For this review, take the finished solid that the model builds, in its own axes (mm). Face numbers are marked on the shaded views. A direction names the side the tool comes from. Coordinates: 2 decimals unless noted, no trailing zeros. Write each loop counter-clockwise with the first axis right and the second up, starting at its lowest first coordinate (ties: lowest second). Pieces come first, ordered by that corner, then holes. Notation, with made-up numbers: M -2,19.5 L 46,19.5 A28 ccw 46,44.5 Z; hole C 61.5,66 d4. An arc over 180 degrees is marked long. One line per question, with ' | ' between items.
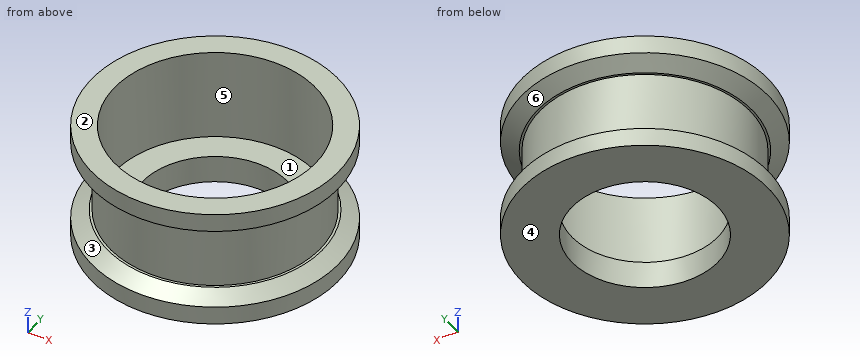
from build123d import *

# Parameters (mm, degrees)
SKETCH1_R           = 13.5
SKETCH1_R_2         = 8
BOSS_EXTRUDE1_DEPTH = 13
SKETCH2_R           = 11
CUT_EXTRUDE1_DEPTH  = 10
CUT_EXTRUDE2_START  = -3
SKETCH3_OUTSIDE_W   = 37.068
SKETCH3_OUTSIDE_H   = 37.068
SKETCH3_OUTSIDE_R   = 11.5
CUT_EXTRUDE2_DEPTH  = 7
CHAMFER1_SIZE       = 1.75
CHAMFER1_SIZE2      = 1.010362971
CHAMFER2_SIZE       = 1
CHAMFER2_SIZE2      = 1.732050808


with BuildPart() as part:
    # Sketch1 → Boss-Extrude1 (new body)
    with BuildSketch(Plane.XY):
        Circle(SKETCH1_R)
        Circle(SKETCH1_R_2, mode=Mode.SUBTRACT)
    extrude(amount=BOSS_EXTRUDE1_DEPTH)

    # Sketch2 → Cut-Extrude1 (cut)
    with BuildSketch(Plane.XY.offset(13)):
        Circle(SKETCH2_R)
    extrude(amount=-CUT_EXTRUDE1_DEPTH, mode=Mode.SUBTRACT)

    # Sketch3 outside → Cut-Extrude2 (cut)
    with BuildSketch(Plane.XY.offset(13).offset(CUT_EXTRUDE2_START)):
        Rectangle(SKETCH3_OUTSIDE_W, SKETCH3_OUTSIDE_H)
        Circle(SKETCH3_OUTSIDE_R, mode=Mode.SUBTRACT)
    extrude(amount=-CUT_EXTRUDE2_DEPTH, mode=Mode.SUBTRACT)

    # Chamfer1
    chamfer1_edges = [part.edges().sort_by_distance(p)[0] for p in [
        (-13.5, 0, 10),
    ]]
    chamfer1_side = [part.faces().sort_by_distance(p)[0] for p in [
        (-13.118162338, 0, 10),
    ]]
    chamfer(chamfer1_edges, length=CHAMFER1_SIZE, length2=CHAMFER1_SIZE2, reference=chamfer1_side[0])

    # Chamfer2
    chamfer2_edges = [part.edges().sort_by_distance(p)[0] for p in [
        (-13.5, 0, 3),
    ]]
    chamfer2_side = [part.faces().sort_by_distance(p)[0] for p in [
        (-13.5, 0, 1.5),
    ]]
    chamfer(chamfer2_edges, length=CHAMFER2_SIZE, length2=CHAMFER2_SIZE2, reference=chamfer2_side[0])


solid = part.part
1. Take a section at C-C on z = 4.5. State the section outline as (x, y) points.
Computed values:
outline: C 0,0 d23; hole C 0,0 d22
2. Machinability: for the marked faces 4, 5 and 6, which of the approach directions +Z, -Z, +X, -X, +Y, -Y give a long, thin tool a straight path to every point of the face, cutting with its end or side? Answer none if there is none.
Computed values:
face 4: -Z, +X, -X, +Y, -Y | face 5: +Z | face 6: none
3. Draft analysis for pull direction X (two halves, no side actions). For the marked faces 1, 2 and 3, state which applies: pulls with the +X half, pulls with the -X half, needs draft (parallel to the pull), parting line crosses it, or undercut.
Computed values:
face 1: undercut | face 2: needs draft | face 3: parting line crosses it
4. For line 1 along X through (y, z) = (0, 0.8); line 2 along Y through (x, z) = (0.25, 11.5), list the stretches that pass through material, from the lowest coordinate up.
Computed values:
line 1: x = -13.5 to -8, 8 to 13.5 | line 2: y = -13.5 to -11, 11 to 13.5
5. Clearance check with flat-ended pins moving along their axes: P1, Ø1, axis at x = -2.5, z = 4.5, coming from the +Y side; P2, Ø2, axis at x = -5.5, y = 3, coming from the -Z side; P3, Ø12, axis at x = 4, y = -5, coming from the -Z side; P4, Ø2, axis at y = -9, z = 8, coming from the +X side. State where each tip first meets the part, or that it passes through.
Computed values:
P1: stops at y = 11.32 | P2: passes through | P3: stops at z = 0 | P4: stops at x = 8.26
6. Take a section at A-A on x = 0. State the section outline as (y, z) points.
Computed values:
outline: M -13.5,0 L -8,0 L -8,3 L -11,3 L -11,13 L -13.5,13 L -13.5,11.01 L -11.75,10 L -11.5,10 L -11.5,3 L -11.77,3 L -13.5,2 Z; M 8,0 L 13.5,0 L 13.5,2 L 11.77,3 L 11.5,3 L 11.5,10 L 11.75,10 L 13.5,11.01 L 13.5,13 L 11,13 L 11,3 L 8,3 Z
7. Take a section at D-D on z = 12.25. State the section outline as (x, y) points, plus the area to 3 significant figures.
Computed values:
outline: C 0,0 d27; hole C 0,0 d22 | area: 192 mm2
